Autodesk Inventor part; units mm, degrees
ref_plane "YZ Plane" through (0, 0, 0) normal (1, 0, 0) x (0, 1, 0)
ref_plane "XZ Plane" through (0, 0, 0) normal (0, 1, 0) x (-1, 0, 0)
ref_plane "XY Plane" through (0, 0, 0) normal (0, 0, 1) x (1, 0, 0)
sketch "Sketch1" plane through (0, 0, 0) normal (0, 0, 1) x (1, 0, 0)
  line L0 (-30, -30) -> (30, -30)
  line L1 (30, -30) -> (30, 30)
  line L2 (30, 30) -> (-30, 30)
  line L3 (-30, 30) -> (-30, -30)
  line L4 (-30, -30) -> (30, 30) construction
  line L5 (30, -30) -> (-30, 30) construction
  point P0 (0, 0)
  dimension "d0" = 60
  dimension "d1" = 60
extrude "Extrusion1" add sketch "Sketch1" along normal blind 43
sketch "Sketch2" plane through (0, 0, 43) normal (0, 0, 1) x (1, 0, 0)
  circle A0 centre (0, 0) radius 18
  dimension "d4" = 36
extrude "Extrusion2" cut sketch "Sketch2" against normal blind 43
sketch "Sketch3" plane through (30, -30, 0) normal (1, 0, 0) x (0, 0, -1)
  line L0 (0, 0) -> (0, 60)
  line L1 (0, 60) -> (-43, 60)
  line L2 (-43, 0) -> (-43, 60)
  line L3 (0, 0) -> (-43, 0)
  circle A0 centre (-21.5, 30) radius 15
  point P0 (0, 30)
  dimension "d7" = 30
  dimension "d8" = 21.5
  dimension "d9" = 30
  dimension "d10" = 60
  dimension "d11" = 43
extrude "Extrusion3" cut sketch "Sketch3" against normal blind 430 contours A0
sketch "Sketch4" plane through (-30, 30, 0) normal (0, 1, 0) x (1, 0, 0)
  line L0 (60, 0) -> (0, 0)
  line L1 (0, 0) -> (0, -43)
  line L2 (60, -43) -> (0, -43)
  line L3 (60, 0) -> (60, -43)
  circle A0 centre (30, -21.5) radius 20.5
  point P0 (30, 0)
  dimension "d14" = 41
  dimension "d15" = 60
  dimension "d16" = 43
  dimension "d17" = 21.5
  dimension "d18" = 30
extrude "Extrusion4" cut sketch "Sketch4" against normal blind 430 contours A0
sketch "Sketch5" plane through (0, 0, 43) normal (0, 0, 1) x (1, 0, 0)
  circle A0 centre (0, 0) radius 18
  line L0 (-30, -30) -> (30, -30)
  line L1 (30, -30) -> (30, 30)
  line L2 (30, 30) -> (-30, 30)
  line L3 (-30, 30) -> (-30, -30)
  circle A1 centre (0, 0) radius 20
  dimension "d21" = 2
extrude "Extrusion5" add sketch "Sketch5" along normal blind 10 contours A1
sketch "Sketch6" plane through (0, 0, 43) normal (0, 0, 1) x (1, 0, 0)
  circle A0 centre (0, 0) radius 20
  line L0 (-30, -30) -> (30, -30)
  line L1 (30, -30) -> (30, 30)
  line L2 (30, 30) -> (-30, 30)
  line L3 (-30, 30) -> (-30, -30)
  circle A1 centre (-26, -26) radius 1.75
  dimension "d24" = 3.5
  dimension "d25" = 4
  dimension "d26" = 4
extrude "Extrusion6" cut sketch "Sketch6" against normal blind 500 contours A1
pattern_circular "Circular Pattern1" count 4 over 360 about axis through (0, 0, 43) along (0, 0, -1) of "Extrusion6"
sketch "Sketch7" plane through (0, 0, 0) normal (0, 0, -1) x (-1, 0, 0)
  circle A0 centre (-26, -26) radius 1.75
  circle A1 centre (-26, 26) radius 1.75
  circle A2 centre (26, 26) radius 1.75
  circle A3 centre (26, -26) radius 1.75
  circle A4 centre (0, 0) radius 18
  line L0 (30, -30) -> (-30, -30)
  line L1 (30, 30) -> (30, -30)
  line L2 (-30, 30) -> (30, 30)
  line L3 (-30, -30) -> (-30, 30)
  line L4 (49.4282, -48.51) -> (-49.4282, -48.51)
  line L5 (-49.4282, -48.51) -> (-49.4282, 48.51)
  line L6 (-49.4282, 48.51) -> (49.4282, 48.51)
  line L7 (49.4282, 48.51) -> (49.4282, -48.51)
  line L8 (49.4282, -48.51) -> (-49.4282, 48.51) construction
  line L9 (-49.4282, -48.51) -> (49.4282, 48.51) construction
extrude "Extrusion7" cut sketch "Sketch7" against normal blind 21.5 contours A0 | A1 | A2 | A3 | A4 | L0 L3 L2 L1 | L4 L5 L6 L7
sketch "Sketch13" plane through (0, 0, 43) normal (0, 0, 1) x (1, 0, 0)
  circle A0 centre (0, 0) radius 20
  line L0 (-30, -30) -> (30, -30)
  line L1 (30, -30) -> (30, 30)
  line L2 (30, 30) -> (-30, 30)
  line L3 (-30, 30) -> (-30, -30)
  circle A1 centre (0, 0) radius 30
  dimension "d55" = 10
equation "\"d8\" = 0.5 * d11"
equation "\"d9\" = 0.5 * d10"
equation "\"d17\" = 0.5 * d16"
equation "\"d18\" = 0.5 * d15"
equation "\"d26\" = d25"
equation "\"d32\" = 0.5 * d2"
properties part number "peca2"
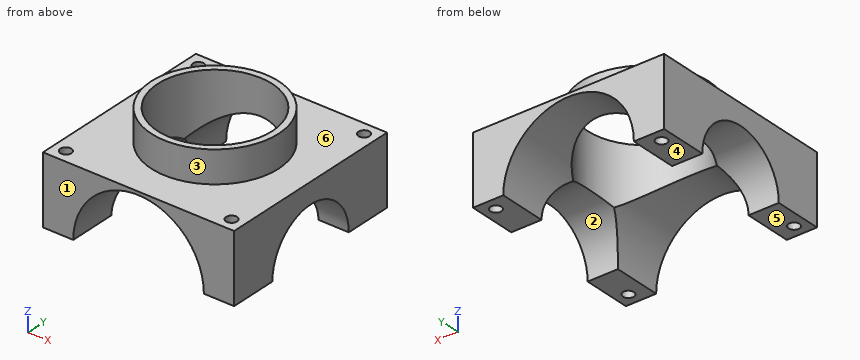
Verification items for the finished model (mm, model axes). Face numbers are marked on the shaded views. A direction names the side the tool comes from. Round coordinates to 2 decimals unless told otherwise and drop trailing zeros. Loops run counter-clockwise (first coordinate to the right, second up) from the corner with the lowest first, then second, coordinate; pieces in that order, holes last. Notation, with made-up numbers: (28.5, 44) - (72.5, 44) arc R23 cw to (72.5, 55) - close; hole circle Ø6 at (25, 9). An arc over 180 degrees is marked (long way). Answer in a Markdown table with one row per item. Add a question column.
Q1. Section check A-A on y = 0. Enter the section's corners in (x, z), plus the area to 3 significant figures.
Q2. Material ranges on line 1 (Y direction, x = 26, z = 34); line 2 (X direction, y = -25.5, z = 39); line 3 (X direction, y = 17, z = 26), recorded low to high.
Q3. Gauge pin test, flat end, axial feed: pin 1 (12 mm diameter, centred on x = 16.5, y = 24, fed in from +Z). Record the tip position at first contact, or that the pin passes through.
Q4. Release check for a two-part mould opening along Y. For the marked faces 1, 2, 3 and 4 record: pulls with the +Y half, pulls with the -Y half, needs draft (parallel to the pull), parting line crosses it, or undercut.
Q5. Section check B-B on x = 0. Enter the section's corners in (y, z), plus the area to 3 significant figures.
Q6. Tool access check on the marked faces 5 and 6. Record the directions out of +Z, -Z, +X, -X, +Y, -Y that give a thin tool (end or side, any length) a straight path to the whole face; none if there is none.
Q7. Section check D-D on y = 26. Enter the section's corners in (x, z).
Q8. Section check C-C on x = -26. Enter the section's corners in (y, z), plus the area to 3 significant figures.
Found:
| question | item | result |
|---|---|---|
| 1 | outline | (-30, 36.5) - (-18, 36.5) - (-18, 53) - (-20, 53) - (-20, 43) - (-30, 43) - close; (18, 36.5) - (30, 36.5) - (30, 43) - (20, 43) - (20, 53) - (18, 53) - close |
| 1 | area | 196 mm² |
| 2 | line 1 | y = -30 to -27.75, -24.25 to -8.29, 8.29 to 24.25, 27.75 to 30 |
| 2 | line 2 | x = -30 to -27.68, -24.32 to -10.68, 10.68 to 24.32, 27.68 to 30 |
| 2 | line 3 | x = -30 to -20, 20 to 30 |
| 3 | pin 1 | stops at z = 43 |
| 4 | face 1 | pulls with the -Y half |
| 4 | face 2 | undercut |
| 4 | face 3 | parting line crosses it |
| 4 | face 4 | needs draft |
| 5 | outline | (-30, 42) - (-18, 42) - (-18, 53) - (-20, 53) - (-20, 43) - (-30, 43) - close; (18, 42) - (30, 42) - (30, 43) - (20, 43) - (20, 53) - (18, 53) - close |
| 5 | area | 64.0 mm² |
| 6 | face 5 | -Z, +X, -X, +Y, -Y |
| 6 | face 6 | +Z |
| 7 | outline | (-30, 21.5) - (-27.75, 21.5) - (-27.75, 43) - (-30, 43) - close; (-24.25, 21.5) - (-20.5, 21.5) arc R20.5 cw to (20.5, 21.5) - (24.25, 21.5) - (24.25, 43) - (-24.25, 43) - close; (27.75, 21.5) - (30, 21.5) - (30, 43) - (27.75, 43) - close |
| 8 | outline | (-30, 21.5) - (-27.75, 21.5) - (-27.75, 43) - (-30, 43) - close; (-24.25, 21.5) - (-15, 21.5) arc R15 cw to (15, 21.5) - (24.25, 21.5) - (24.25, 43) - (-24.25, 43) - close; (27.75, 21.5) - (30, 21.5) - (30, 43) - (27.75, 43) - close |
| 8 | area | 786 mm² |
